Input: part model. Units: mm. Frame: model coordinates. A direction names the side the tool comes from. Coordinates: 2 decimals unless noted, no trailing zeros. Order: outer loops, then holes, each group sorted by start corner. A loop starts at its lowest first (then second) coordinate and runs counter-clockwise, first axis right, second up. Notation, with made-up numbers: (32, -26) -> (43, -26) arc R22 cw to (43, -17) -> close; hole circle Ø1 at (48.5, -1). An arc over 180 degrees is marked (long way). Use one line per item in the form item = value. Start each with the question number.
1) Section query B-B on y = 0.65. Count the separate pieces of the cut face and the enclosed holes in it, then the cut area to 3 significant figures.
2) Ray query, line 1 along Z through (x, y) = (18, 1.3); line 2 along Y through (x, z) = (11.5, 1); line 3 along Z through (x, y) = (12.45, 1.4). Return the intervals inside material, ascending.
3) Section query A-A on x = 31.2. Output: boundary loops of the cut face in (y, z).
4) Section query C-C on y = 4.05. Output: boundary loops of the cut face in (x, z) (3 decimals).
5) Access query for faces 4 (the cylindrical face through (1.55, 1.23, -0.03)), 5 (the flat face through (19.9, 1, 6)), 6 (the flat face through (19.9, 1, -6)). Directions: +Z, -Z, +X, -X, +Y, -Y. A direction counts if a zero-diameter tool reaches every point of the face in a straight line with its end or side. Return the directions, or none.
6) Pin query (flat end, axial travel): pin 1 (2 mm diameter, centred on y = 1.5, z = -6.5, fed in from -X); pin 2 (1 mm diameter, centred on x = 21.5, y = 1.5, fed in from -Z); pin 3 (5.5 mm diameter, centred on x = 26, z = 3.5, fed in from +Y); pin 4 (0.8 mm diameter, centred on x = 9.9, z = 0, fed in from +Y). Return the tip coordinate at first contact, or that it passes through.
7) Draft query along Z for faces 1 (the flat face through (20, 5, 2)), 2 (the flat face through (26.922, 1.232, -2.846)), 3 (the cylindrical face through (24.218, 1.232, -0.21)). Return one class per face: pulls with the +Z half, pulls with the -Z half, needs draft (parallel to the pull), parting line crosses it, or undercut.
from build123d import *

# Parameters (mm, degrees)
SKETCH6_R           = 0.7
BOSS_EXTRUDE3_DEPTH = 2.5
SKETCH7_R           = 3.625
BOSS_EXTRUDE4_DEPTH = 2.5
SKETCH8_R           = 2.175
CUT_EXTRUDE3_DEPTH  = 3.4
CUT_EXTRUDE4_REACH  = 3.6
SKETCH9_R           = 1.25


with BuildPart() as part:
    # Sketch6 → Boss-Extrude3 (new body)
    with BuildSketch(Plane(origin=(0, 0, 0), x_dir=(1, 0, 0), z_dir=(0, 1, 0))):
        with BuildLine():
            Line((16.1, 7.6), (16.1, 3.459126984))
            Line((16.1, 3.459126984), (2.25, 2.25))
            ThreePointArc((2.25, 2.25), (0, 0), (2.25, -2.25))
            Line((2.25, -2.25), (16.1, -3.459126984))
            Line((16.1, -3.459126984), (16.1, -7.6))
            ThreePointArc((16.1, -7.6), (18, -9.5), (19.9, -7.6))
            Line((19.9, -7.6), (19.9, -3.459126984))
            Line((19.9, -3.459126984), (33.75, -2.25))
            ThreePointArc((33.75, -2.25), (36, 0), (33.75, 2.25))
            Line((33.75, 2.25), (19.9, 3.459126984))
            Line((19.9, 3.459126984), (19.9, 7.6))
            ThreePointArc((19.9, 7.6), (18, 9.5), (16.1, 7.6))
        make_face()
        with Locations((33.75, 0)):
            Circle(SKETCH6_R, mode=Mode.SUBTRACT)
        with Locations((31.2, 0)):
            Circle(SKETCH6_R, mode=Mode.SUBTRACT)
        with Locations((28.65, 0)):
            Circle(SKETCH6_R, mode=Mode.SUBTRACT)
        with Locations((26.1, 0)):
            Circle(SKETCH6_R, mode=Mode.SUBTRACT)
        with Locations((23.55, 0)):
            Circle(SKETCH6_R, mode=Mode.SUBTRACT)
        with Locations((18, -7.6)):
            Circle(SKETCH6_R, mode=Mode.SUBTRACT)
        with Locations((18, -5.2)):
            Circle(SKETCH6_R, mode=Mode.SUBTRACT)
        with Locations((12.45, 0)):
            Circle(SKETCH6_R, mode=Mode.SUBTRACT)
        with Locations((9.9, 0)):
            Circle(SKETCH6_R, mode=Mode.SUBTRACT)
        with Locations((7.35, 0)):
            Circle(SKETCH6_R, mode=Mode.SUBTRACT)
        with Locations((4.8, 0)):
            Circle(SKETCH6_R, mode=Mode.SUBTRACT)
        with Locations((2.25, 0)):
            Circle(SKETCH6_R, mode=Mode.SUBTRACT)
        with Locations((18, 5.2)):
            Circle(SKETCH6_R, mode=Mode.SUBTRACT)
        with Locations((18, 7.6)):
            Circle(SKETCH6_R, mode=Mode.SUBTRACT)
    extrude(amount=BOSS_EXTRUDE3_DEPTH)

    # Sketch7 → Boss-Extrude4 (add)
    with BuildSketch(Plane(origin=(0, 2.5, 0), x_dir=(1, 0, 0), z_dir=(0, 1, 0))):
        with Locations((18, 0)):
            Circle(SKETCH7_R)
    extrude(amount=BOSS_EXTRUDE4_DEPTH)

    # Sketch8 → Cut-Extrude3 (cut)
    with BuildSketch(Plane(origin=(0, 5, 0), x_dir=(1, 0, 0), z_dir=(0, 1, 0))):
        with Locations((18, 0)):
            Circle(SKETCH8_R)
    extrude(amount=-CUT_EXTRUDE3_DEPTH, mode=Mode.SUBTRACT)

    # Sketch9 → Cut-Extrude4 (cut, up to next)
    with BuildSketch(Plane(origin=(0, 1.6, 0), x_dir=(1, 0, 0), z_dir=(0, 1, 0)), mode=Mode.PRIVATE) as cut_extrude4_sk1:
        with Locations((18, 0)):
            Circle(SKETCH9_R)
    cut_extrude4_tool1 = extrude(cut_extrude4_sk1.sketch, amount=-CUT_EXTRUDE4_REACH, mode=Mode.PRIVATE) & part.part
    add(cut_extrude4_tool1.solids().sort_by_distance((18, 1.6, 0))[0], mode=Mode.SUBTRACT)


solid = part.part
Answers below:
q1.separate_pieces = 1
q1.enclosed_holes = 15
q1.area = 217 mm^2
q2.line_1 = -9.5 to -8.3, -6.9 to -5.9, -4.5 to -1.25, 1.25 to 4.5, 5.9 to 6.9, 8.3 to 9.5
q2.line_2 = 0 to 2.5
q2.line_3 = -3.14 to -0.7, 0.7 to 3.14
q3.outline = (0, -2.47) -> (2.5, -2.47) -> (2.5, -0.7) -> (0, -0.7) -> close; (0, 0.7) -> (2.5, 0.7) -> (2.5, 2.47) -> (0, 2.47) -> close
q4.outline = circle Ø7.25 at (18, 0); hole circle Ø4.35 at (18, 0)
q5.face_4 = +Y, -Y
q5.face_5 = +Z, +X, +Y, -Y
q5.face_6 = -Z, +X, +Y, -Y
q6.pin_1 = 16.1
q6.pin_2 = -3.36
q6.pin_3 = 2.5
q6.pin_4 = through
q7.face_1 = needs draft
q7.face_2 = pulls with the -Z half
q7.face_3 = undercut
